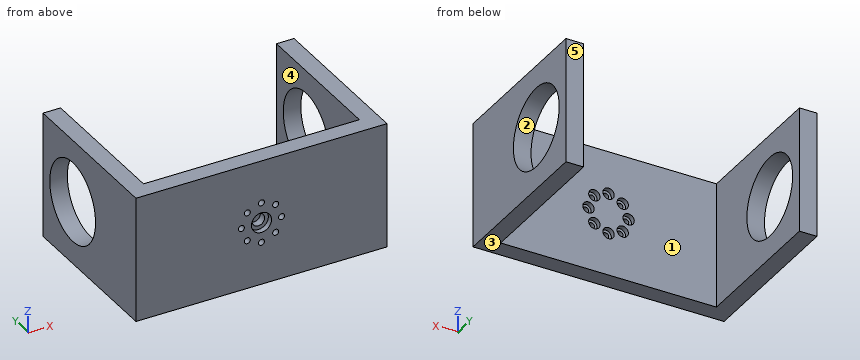
from build123d import *

# Parameters (mm, degrees)
BOSS_EXTRUDE1_DEPTH                             = 50
CBORE_FOR_M2_SOCKET_HEAD_CAP_SCREW1_D           = 2.4
CBORE_FOR_M2_SOCKET_HEAD_CAP_SCREW1_CBORE_D     = 4.5
CBORE_FOR_M2_SOCKET_HEAD_CAP_SCREW1_CBORE_DEPTH = 2
SKETCH7_R                                       = 4
CUT_EXTRUDE2_DEPTH                              = 2.2
SKETCH8_R                                       = 2.5
CUT_EXTRUDE3_DEPTH                              = 3
CUT_EXTRUDE4_DEPTH                              = 124.991935222
CUT_EXTRUDE4_DEPTH_BACK                         = 124.991935222
SKETCH3_R                                       = 16


with BuildPart() as part:
    # Sketch1 → Boss-Extrude1 (new body)
    with BuildSketch(Plane.XY):
        Polygon((-50, 0), (50, 0), (50, 65), (43, 65), (43, 7), (-43, 7), (-43, 65), (-50, 65), align=None)
    extrude(amount=BOSS_EXTRUDE1_DEPTH)

    # CBORE for M2 Socket Head Cap Screw1 (through all)
    with Locations(Plane(origin=(0, 7, 17), x_dir=(0, 0, 1), z_dir=(0, 1, 0))):
        with Locations((0, 0), (2.343145751, 5.656854249), (8, 8), (13.656854249, 5.656854249), (16, 0), (13.656854249, -5.656854249), (8, -8), (2.343145751, -5.656854249)):
            CounterBoreHole(CBORE_FOR_M2_SOCKET_HEAD_CAP_SCREW1_D / 2, CBORE_FOR_M2_SOCKET_HEAD_CAP_SCREW1_CBORE_D / 2, CBORE_FOR_M2_SOCKET_HEAD_CAP_SCREW1_CBORE_DEPTH)

    # Sketch7 → Cut-Extrude2 (cut)
    with BuildSketch(Plane.XZ):
        with Locations(Location((0, 25, 0), (0, 0, 270))):
            Circle(SKETCH7_R)
    extrude(amount=-CUT_EXTRUDE2_DEPTH, mode=Mode.SUBTRACT)

    # Sketch8 → Cut-Extrude3 (cut)
    with BuildSketch(Plane.XZ.offset(-2.2)):
        with Locations(Location((0, 25, 0), (0, 0, 270))):
            Circle(SKETCH8_R)
    extrude(amount=-CUT_EXTRUDE3_DEPTH, mode=Mode.SUBTRACT)

    # Sketch3 → Cut-Extrude4 (cut, two sides: drawn at the far end of the back side and taken through both)
    with BuildSketch(Plane(origin=(43, 0, 0), x_dir=(0, 0, -1), z_dir=(1, 0, 0)).offset(-CUT_EXTRUDE4_DEPTH_BACK)):
        with Locations(Location((-25, 44.25, 0), (0, 0, 90))):
            Circle(SKETCH3_R)
    extrude(amount=CUT_EXTRUDE4_DEPTH + CUT_EXTRUDE4_DEPTH_BACK, mode=Mode.SUBTRACT)


solid = part.part
CAD build for the part. Positions are in the model's coordinates, mm. Face numbers are marked on the shaded views. A direction names the side the tool comes from. Round coordinates to 2 decimals unless told otherwise and drop trailing zeros. Loops run counter-clockwise (first coordinate to the right, second up) from the corner with the lowest first, then second, coordinate; pieces in that order, holes last.
(1) Cut at B-B (y = 16). Give the cut face in (x, z), plus the area to 3 significant figures.
(2) Cut at A-A (y = 44.25). Give the cut face in (x, z), plus the area to 3 significant figures.
(3) Which spindle directions (+Z, -Z, +X, -X, +Y, -Y) get a long thin tool onto all of the face, cutting with end or side? Do the marked faces 4 and 5. Say none if no direction does.
(4) Wall check: line 1 along X through (y, z) = (3.2, 25); line 2 along Z through (x, y) = (48, 44); line 3 along X through (y, z) = (6, 33). Give the ranges that are in metal, low to high.
(5) Drop flat-ended pins along their axis: pin 1 (2.5 mm diameter, centred on x = 5.66, z = 19.34, fed in from +Y); pin 2 (12 mm diameter, centred on x = 13, z = 37.5, fed in from -Y); pin 3 (3.5 mm diameter, centred on x = 1, z = 16.5, fed in from +Y); pin 4 (2.5 mm diameter, centred on x = 0.5, z = 26, fed in from -Y). Give the stop position or say it passes through.
(6) Cut at D-D (z = 25). State how many separate pieces and enclosed holes the cut face has, plus the area to 3 significant figures.
(7) Cut at C-C (x = 0). Give the cut face in (y, z).
(8) Two-plate mould, pull along Y, no slides. Class the marked faces 1, 2 and 3: +Y half, -Y half, draft (parallel to the pull), parting line (faces both ways), or undercut.
Findings below:
1. outline: (-50, 0) - (-43, 0) - (-43, 50) - (-50, 50) - close; (43, 0) - (50, 0) - (50, 50) - (43, 50) - close
1. area: 700 mm2
2. outline: (-50, 0) - (-43, 0) - (-43, 9) - (-50, 9) - close; (-50, 41) - (-43, 41) - (-43, 50) - (-50, 50) - close; (43, 0) - (50, 0) - (50, 9) - (43, 9) - close; (43, 41) - (50, 41) - (50, 50) - (43, 50) - close
2. area: 252 mm2
3. face 4: +Z, -Z, +Y
3. face 5: +Z, -Z, +X, -X, +Y
4. line 1: x = -50 to -9.2, -6.8 to -2.5, 2.5 to 6.8, 9.2 to 50
4. line 2: z = 0 to 9, 41 to 50
4. line 3: x = -50 to -2.25, 2.25 to 50
5. pin 1: stops at y = 5
5. pin 2: stops at y = 0
5. pin 3: stops at y = 7
5. pin 4: stops at y = 5.2
6. separate pieces: 5
6. enclosed holes: 0
6. area: 989 mm2
7. outline: (0, 0) - (7, 0) - (7, 14.75) - (5, 14.75) - (5, 15.8) - (0, 15.8) - close; (0, 18.2) - (5, 18.2) - (5, 19.25) - (7, 19.25) - (7, 30.75) - (5, 30.75) - (5, 31.8) - (0, 31.8) - (0, 29) - (2.2, 29) - (2.2, 27.5) - (5.2, 27.5) - (5.2, 22.5) - (2.2, 22.5) - (2.2, 21) - (0, 21) - close; (0, 34.2) - (5, 34.2) - (5, 35.25) - (7, 35.25) - (7, 50) - (0, 50) - close
8. face 1: +Y half
8. face 2: undercut
8. face 3: draft
